```python
from build123d import *


with BuildPart() as part:
    # Sketch2 → Revolve1 (revolve)
    with BuildSketch(Plane.XY, mode=Mode.PRIVATE) as revolve1_sk:
        with BuildLine():
            Line((0, 26.9875), (76.2, 26.9875))
            Line((76.2, 26.9875), (0, 41.275))
            Line((0, 41.275), (0, 38.1))
            Line((0, 38.1), (-45.72, 38.1))
            Line((-45.72, 38.1), (-45.72, 34.925))
            Line((-45.72, 34.925), (-2.665476758, 25.68286532))
            ThreePointArc((-2.665476758, 25.68286532), (-1.340221916, 25.470914316), (0, 25.4))
            Line((0, 25.4), (0, 26.9875))
        make_face()
    revolve(revolve1_sk.sketch.rotate(Axis((109.22, 0, 0), (-1, 0, 0)), 90), axis=Axis((109.22, 0, 0), (-1, 0, 0)))


solid = part.part
```
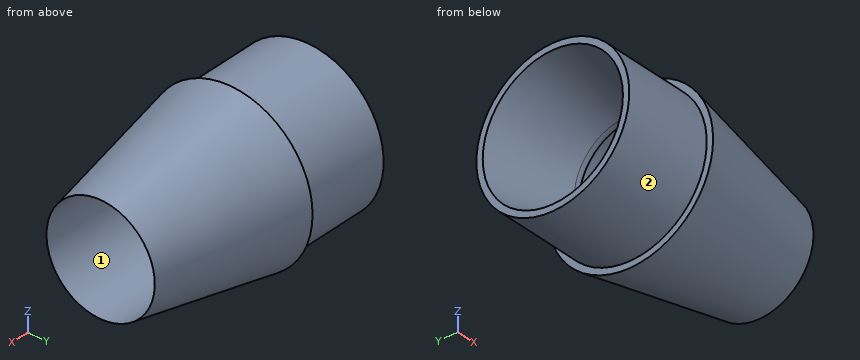
Model file for the job. Use its own axes, mm. Face numbers are marked on the shaded views. Give positions to 0.01 mm unless a question says otherwise; leave off trailing zeros. Loops run counter-clockwise (first coordinate to the right, second up) from the corner with the lowest first, then second, coordinate; pieces in that order, holes last. Notation, with made-up numbers: (-15.75, 23.25) -> (29.25, 23.25) arc R8 cw to (29.25, 36.25) -> close; hole circle Ø4 at (3.25, 80.25). An arc over 180 degrees is marked (long way). Write each question's results on one line, items separated by ' | '.
(1) Cut at C-C on x = -37. List the corners of the cut face in (y, z).
Geometry results:
outline: circle Ø76.2 at (0, 0); hole circle Ø66.11 at (0, 0)
(2) Flat gauge pins, fed straight in: pin 1 Ø1 at (x, z) = (56.5, 28.5) entering from -Y; pin 2 Ø5 at (x, z) = (61, 9) entering from +Y; pin 3 Ø5 at (x, y) = (-27, 30.5) entering from +Z. Where does each tip first touch, or does it go through?
Geometry results:
pin 1: stops at y = -12.57 | pin 2: stops at y = 29.29 | pin 3: stops at z = 25.84
(3) Pull direction Y, two halves, no side cores. Call the marked faces 1 and 2: released by +Y, released by -Y, zero draft, split by the parting line, or undercut.
Geometry results:
face 1: undercut | face 2: split by the parting line
(4) Probe line 1 along Y through (x, z) = (45, 0); line 2 along Y through (x, z) = (-28, 14); line 3 along Z through (x, y) = (-15, 15). List the from-to ranges inside material, lowest first.
Geometry results:
line 1: y = -32.84 to -26.99, 26.99 to 32.84 | line 2: y = -35.43 to -27.79, 27.79 to 35.43 | line 3: z = -35.02 to -24.03, 24.03 to 35.02
(5) Cut at A-A on z = 0. List the corners of the cut face in (x, y) (1 decimal).
Geometry results:
outline: (-45.7, -38.1) -> (0, -38.1) -> (0, -41.3) -> (76.2, -27) -> (0, -27) -> (0, -25.4) arc R12.7 ccw to (-2.7, -25.7) -> (-45.7, -34.9) -> close; (-45.7, 34.9) -> (-2.7, 25.7) arc R12.7 ccw to (0, 25.4) -> (0, 27) -> (76.2, 27) -> (0, 41.3) -> (0, 38.1) -> (-45.7, 38.1) -> close
